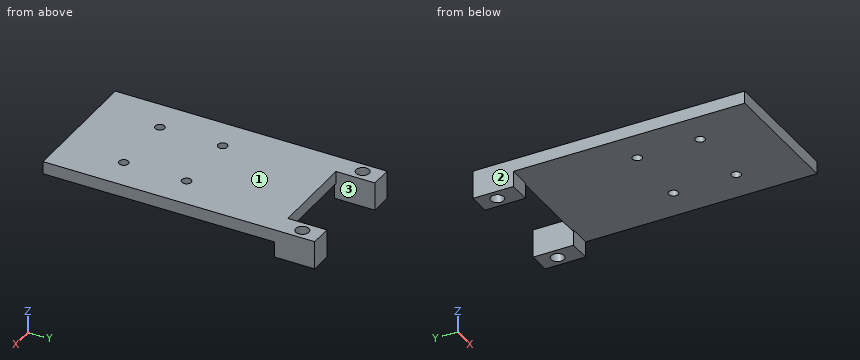
```python
from build123d import *

# Parameters (mm, degrees)
SALIENTE_EXTRUIR1_DEPTH = 4
CROQUIS2_W              = 7
CROQUIS2_H              = 12.866645138
SALIENTE_EXTRUIR2_DEPTH = 5
CROQUIS3_R              = 2.1
CORTAR_EXTRUIR1_DEPTH   = 10
CROQUIS4_R              = 1.5
CORTAR_EXTRUIR2_DEPTH   = 10
CROQUIS5_R              = 1.5
CORTAR_EXTRUIR3_DEPTH   = 10


with BuildPart() as part:
    # Croquis1 → Saliente-Extruir1 (new body)
    with BuildSketch(Plane.XY):
        Polygon((31.808893405, -1059.380585752), (31.808893405, -1140.619885182), (-10.106831803, -1140.619885182), (-10.106831803, -1059.380585752), (-10.106831803, -1054.003240044), (-3.106831803, -1054.003240044), (-3.106831803, -1066.423001802), (24.808893405, -1066.423001802), (24.808893405, -1054.003240044), (31.808893405, -1054.003240044), align=None)
    extrude(amount=SALIENTE_EXTRUIR1_DEPTH)

    # Croquis2 → Saliente-Extruir2 (add)
    with BuildSketch(Plane(origin=(0, 0, 0), x_dir=(-1, 0, 0), z_dir=(0, 0, -1))):
        with Locations((6.606831803, -1060.436562613)):
            Rectangle(CROQUIS2_W, CROQUIS2_H)
        with Locations((-28.308893405, -1060.436562613)):
            Rectangle(CROQUIS2_W, CROQUIS2_H)
    extrude(amount=SALIENTE_EXTRUIR2_DEPTH)

    # Croquis3 → Cortar-Extruir1 (cut)
    with BuildSketch(Plane.XY.offset(4)):
        with Locations((-6.691106595, -1059.869885182)):
            Circle(CROQUIS3_R)
        with Locations((28.308893405, -1059.869885182)):
            Circle(CROQUIS3_R)
    extrude(amount=-CORTAR_EXTRUIR1_DEPTH, mode=Mode.SUBTRACT)

    # Croquis4 → Cortar-Extruir2 (cut)
    with BuildSketch(Plane.XY.offset(4)):
        with Locations((21.329962103, -1120.619885182)):
            Circle(CROQUIS4_R)
        with Locations((0.372099499, -1120.619885182)):
            Circle(CROQUIS4_R)
    extrude(amount=-CORTAR_EXTRUIR2_DEPTH, mode=Mode.SUBTRACT)

    # Croquis5 → Cortar-Extruir3 (cut)
    with BuildSketch(Plane.XY.offset(4)):
        with Locations((0.372099499, -1100.615007654)):
            Circle(CROQUIS5_R)
        with Locations((21.329962103, -1100.619885182)):
            Circle(CROQUIS5_R)
    extrude(amount=-CORTAR_EXTRUIR3_DEPTH, mode=Mode.SUBTRACT)


solid = part.part
```
Here's how the part is built. I have some questions about the finished solid (model axes, mm). Face numbers are marked on the shaded views. Coordinates: 2 decimals unless noted, no trailing zeros. Loops run counter-clockwise (first coordinate to the right, second up) from the corner with the lowest first, then second, coordinate; pieces in that order, holes last. Notation, with made-up numbers: (47, 27.25) -> (83, 27.25) arc R23 cw to (83, 53.25) -> close; hole circle Ø11 at (-21, 53.5). An arc over 180 degrees is marked (long way). Return JSON: item names as keys, results as strings.
1) Will these pins go through, and if not, where does the flat tip stop? pin 1 (4 mm diameter, centred on x = 27, z = -2.5, fed in from -Y); pin 2 (5 mm diameter, centred on x = 21.33, y = -1100.62, fed in from -Z); pin 3 (4 mm diameter, centred on x = 17, z = 1.5, fed in from +Y); pin 4 (8 mm diameter, centred on x = -0.5, y = -1120, fed in from +Z).
Results below:
{"pin 1": "y = -1066.87", "pin 2": "z = 0", "pin 3": "y = -1066.42", "pin 4": "z = 4"}
2) Thinking about a two-plate mould opening in X: for the marked faces 1, 2 and 3, which applies, +X half, -X half, draft (parallel to the pull), parting line (faces both ways), or undercut?
Results below:
{"face 1": "draft", "face 2": "-X half", "face 3": "undercut"}
3) I need wall thicknesses on line 1 (X direction, y = -1060, z = 0.5); line 2 (Y direction, x = 21, z = 1.5); line 3 (Z direction, x = 22, y = -1075.5). Which ranges of each line are inside material? Lowest first, please. Write a range as from..to.
Results below:
{"line 1": "-10.11..-8.79, -4.6..-3.11, 24.81..26.21, 30.4..31.81", "line 2": "-1140.62..-1122.08, -1119.16..-1102.08, -1099.16..-1066.42", "line 3": "0..4"}
4) If we section it at B-B, the plane x = 28: Write out the boundary of the cut face in (y, z), then the cut area to 3 significant figures.
Results below:
{"outline": "(-1140.62, 0) -> (-1066.87, 0) -> (-1066.87, -5) -> (-1061.95, -5) -> (-1061.95, 4) -> (-1140.62, 4) -> close; (-1057.79, -5) -> (-1054, -5) -> (-1054, 4) -> (-1057.79, 4) -> close", "area": "373 mm²"}
5) If we section it at C-C, the plane z = -1: Write out the boundary of the cut face in (x, y).
Results below:
{"outline": "(-10.11, -1066.87) -> (-3.11, -1066.87) -> (-3.11, -1054) -> (-10.11, -1054) -> close; (24.81, -1066.87) -> (31.81, -1066.87) -> (31.81, -1054) -> (24.81, -1054) -> close; hole circle Ø4.2 at (-6.69, -1059.87); hole circle Ø4.2 at (28.31, -1059.87)"}
6) If we section it at A-A, the plane y = -1064.5: Write out the boundary of the cut face in (x, z), then the cut area to 3 significant figures.
Results below:
{"outline": "(-10.11, -5) -> (-3.11, -5) -> (-3.11, 4) -> (-10.11, 4) -> close; (24.81, -5) -> (31.81, -5) -> (31.81, 4) -> (24.81, 4) -> close", "area": "126 mm²"}
7) If we section it at D-D, the plane z = 3: Write out the boundary of the cut face in (x, y) (3 decimals).
Results below:
{"outline": "(-10.107, -1140.62) -> (31.809, -1140.62) -> (31.809, -1054.003) -> (24.809, -1054.003) -> (24.809, -1066.423) -> (-3.107, -1066.423) -> (-3.107, -1054.003) -> (-10.107, -1054.003) -> close; hole circle Ø4.2 at (-6.691, -1059.87); hole circle Ø3 at (0.372, -1120.62); hole circle Ø3 at (0.372, -1100.615); hole circle Ø3 at (21.33, -1120.62); hole circle Ø3 at (21.33, -1100.62); hole circle Ø4.2 at (28.309, -1059.87)"}
